Design review of the part built by this model. Coordinates are the model's own, in mm. Face numbers are marked on the shaded views. A direction names the side the tool comes from. Coordinates: 2 decimals unless noted, no trailing zeros. Write each loop counter-clockwise with the first axis right and the second up, starting at its lowest first coordinate (ties: lowest second). Pieces come first, ordered by that corner, then holes. Notation, with made-up numbers: (35, -5) - (62, -5) arc R17 ccw to (62, 22) - close; hole circle Ø1 at (19, 29). An arc over 180 degrees is marked (long way). One line per item, written item: value.
from build123d import *

# Parameters (mm, degrees)
F0_R     = 27
F0_R_2   = 26
F1_DEPTH = 1
F0_R_3   = 22.5
F2_DEPTH = 5
F3_SIZE  = 0.8


with BuildPart() as f1:
    # F0 (on Top) → F1 (new body, symmetric)
    with BuildSketch(Plane.XY):
        Circle(F0_R)
        Circle(F0_R_2, mode=Mode.SUBTRACT)
    extrude(amount=F1_DEPTH, both=True)

    # F0 (on Top) → F2 (join, symmetric)
    with BuildSketch(Plane.XY):
        Circle(F0_R_2)
        Circle(F0_R_3, mode=Mode.SUBTRACT)
    extrude(amount=F2_DEPTH, both=True)

    # F3
    f3_edges = [f1.edges().sort_by_distance(p)[0] for p in [
        (-27, 0, 1),
        (-27, 0, -1),
    ]]
    chamfer(f3_edges, length=F3_SIZE)


solid = f1.part
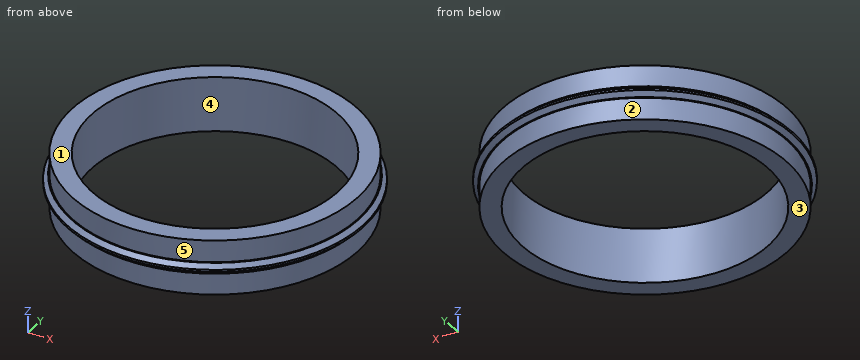
1. Wall thickness on line 1 along Y through (x, z) = (-0.5, -1.5); line 2 along X through (y, z) = (-3.5, 2); line 3 along Y through (x, z) = (10, -4.5): over which ranges is each line inside the solid? List them lowest first.
Answer block:
line 1: y = -26 to -22.49, 22.49 to 26
line 2: x = -25.76 to -22.23, 22.23 to 25.76
line 3: y = -24 to -20.16, 20.16 to 24
2. Consider section C-C, the plane z = 2.25. Write out the cut boundary in (x, y), then the cut area to 3 significant figures.
Answer block:
outline: circle Ø52 at (0, 0); hole circle Ø45 at (0, 0)
area: 533 mm^2
3. Mouldability with a two-part tool opening along X and no side actions: class the marked faces 3, 4 and 5 as released by +X, released by -X, zero draft, split by the parting line, or undercut.
Answer block:
face 3: zero draft
face 4: undercut
face 5: split by the parting line
4. For the marked faces 1 and 2, list the 3-axis set-ups (+Z, -Z, +X, -X, +Y, -Y) from which the entire face can be reached by the end or side of a thin tool; tool diameter is ignored.
Answer block:
face 1: +Z, +X, -X, +Y, -Y
face 2: -Z
5. Consider section A-A, the plane x = 0. Write out the cut boundary in (y, z), then the cut area to 3 significant figures.
Answer block:
outline: (-27, -0.2) - (-26.2, -1) - (-26, -1) - (-26, -5) - (-22.5, -5) - (-22.5, 5) - (-26, 5) - (-26, 1) - (-26.2, 1) - (-27, 0.2) - close; (22.5, -5) - (26, -5) - (26, -1) - (26.2, -1) - (27, -0.2) - (27, 0.2) - (26.2, 1) - (26, 1) - (26, 5) - (22.5, 5) - close
area: 72.7 mm^2
6. Insertion check: pin 1 Ø5 at (x, z) = (-21, -0.5) entering from +Y; pin 2 Ø2 at (y, z) = (18, -3) entering from -X; pin 3 Ø5 at (x, z) = (16.5, -3) entering from +Y. Each pin has a flat end and moves straight along its axis. Give the tip position at first contact, or say it passes through.
Answer block:
pin 1: stops at y = 19.65
pin 2: stops at x = -19.67
pin 3: stops at y = 21.91
